The listing builds one solid part. Answer for the finished solid, in the listing's coordinates (mm). A direction names the side the tool comes from. Coordinates: 2 decimals unless noted, no trailing zeros. Order: outer loops, then holes, each group sorted by start corner. A loop starts at its lowest first (then second) coordinate and runs counter-clockwise, first axis right, second up. Notation, with made-up numbers: (-34, 5) - (-18, 5) arc R9 cw to (-18, 21) - close; hole circle Ø11 at (77, 6.25). An arc over 180 degrees is marked (long way). Use a Markdown table: item, result. Add a question column.
Item 1: The mould has two halves that part along Z. Classify faces 1 (the cylindrical face through (37, -3, 0)), 2 (the flat face through (0, 3.3, 0.1)), 3 (the flat face through (-4.411, 1.268, 2.155)): released by +Z, released by -Z, zero draft, split by the parting line, or undercut.
Item 2: The part is cut by section A-A, the plane x = 19. Give the vertices of the cut face in (y, z).
Item 3: Flat-ended cylindrical pins translate along their axes: P1, Ø1, axis at x = 54, z = -2.5, coming from the -Y side; P2, Ø4, axis at x = 3.5, y = -0.5, coming from the -Z side; P3, Ø3, axis at x = 66, y = 3, coming from the -Z side. Find the tip coordinate at first contact, or state that the pin passes through.
Item 4: For faces 4 (the flat face through (75, 0, 0)), 5 (the flat face through (-4, -2.5, 0)), determine the directions among +Z, -Z, +X, -X, +Y, -Y from which every point of the face is accessible in a straight line to the end or side of a thin tool.
Item 5: Find the intervals of material crossed by line 1 along X through (y, z) = (3, 1.5); line 2 along Z through (x, y) = (35, 0); line 3 along Z through (x, y) = (41.5, 2.25), in increasing order.
Autodesk Inventor part; units mm, degrees
ref_plane "Work Plane1" through (29, 0, 0) normal (0, -1, 0) x (1, 0, 0)
ref_plane "YZ Plane" through (0, 0, 0) normal (1, 0, 0) x (0, 1, 0)
ref_plane "XZ Plane" through (0, 0, 0) normal (0, 1, 0) x (-1, 0, 0)
sketch "Sketch1" plane through (0, 0, 0) normal (0, 0, 1) x (1, 0, 0)
  line L0 (-1.3333, 0) -> (75, 0)
  line L1 (75, 0) -> (75, 3)
  line L2 (75, 3) -> (51, 3)
  line L3 (51, 3) -> (50.3865, 3)
  line L4 (50.3865, 3) -> (0, 3)
  line L5 (0, 3) -> (0, 5)
  line L6 (0, 5) -> (-6, 5)
  line L7 (-6, 5) -> (-6, 2.8868)
  line L8 (-6, 2.8868) -> (-3, 2.8868)
  line L9 (-3, 2.8868) -> (-1.3333, 0)
  line L10 (-22.2, 0) -> (91.2, 0)
  line L11 (0, -1) -> (0, 6)
  line L12 (51, 3) -> (0, 3) construction
  dimension "d1" = 24
  dimension "d2" = 0.6136
  dimension "d3" = 6
  dimension "d4" = 3
  dimension "d5" = 60
  dimension "d6" = 6
  dimension "d7" = 6
  dimension "d8" = 5.7735
  dimension "d9" = 10
  dimension "d26" = 75
revolve "Body" add sketch "Sketch1" angle 360 about axis through (-1.3333, 0, 0) along (1, 0, 0)
sketch "Sketch2" plane through (-6, 0, 0) normal (-1, 0, 0) x (0, 0, 1)
  circle A0 centre (0, 0) radius 2.8868
  line L0 (0, -7) -> (0, 7)
  line L1 (-7, 0) -> (7, 0)
  line L2 (2.8868, 0) -> (1.4434, -2.5)
  line L3 (1.4434, -2.5) -> (-1.4434, -2.5)
  line L4 (-1.4434, -2.5) -> (-2.8868, 0)
  line L5 (-2.8868, 0) -> (-1.4434, 2.5)
  line L6 (-1.4434, 2.5) -> (1.4434, 2.5)
  line L7 (1.4434, 2.5) -> (2.8868, 0)
extrude "Slot" add sketch "Sketch2" against normal up to next contours L7 A0 | A0 L2 | L6 L0 A0 | A0 L0 L3 | L0 L6 A0 | A0 L3 L0 | L4 A0 | A0 L5
fillet "Fillet1" radius 0.4 1 edges at (-6, -5, 0)
thread "Thread"
chamfer "Chamfer1" distance 0.6135 distance2 0.6135 1 edges at (75, -3, 0) measured on face at (75, -0.9709, -1.4067)
ref_plane "Work Plane1" through (29, 0, 0) normal (0, -1, 0) x (1, 0, 0)
fillet "Fillet2" radius 0.1 1 edges at (0, -3, 0)
equation "\"d1\" = GEL"
equation "\"d3\" = KOH"
equation "\"d4\" = INTI"
equation "\"d6\" = GD"
equation "\"d7\" = BDM"
equation "\"d8\" = 1.1547 * SW"
equation "\"d9\" = KOD"
equation "\"d26\" = NLG"
equation "\"d30\" = R"
equation "\"d17\" = RR"
equation "\"d13\" = GEL"
equation "\"d15\" = -0.5 * SPD + 0.5 * GD"
equation "\"d16\" = GUL"
equation "\"GD\" = NND"
equation "\"NLG\" = 75"
equation "\"GEL\" = 24"
equation "\"KOD\" = 10"
equation "\"KOH\" = NND"
equation "\"INTI\" = 3"
equation "\"GAL\" = 0.61345 * PTC"
equation "\"GUL\" = 0.61345 * PTC"
equation "\"BDM\" = NND"
equation "\"SW\" = 5"
equation "\"RR\" = 0.4"
equation "\"SPD\" = NND - 1.2269 * PTC"
equation "\"R\" = 0.1"
equation "\"PHH\" = 0.1 * NND"
equation "\"GD1\" = THREADDIA - 1.2269 * PTC"
equation "\"THREADDIA\" = 6"
equation "\"FAWI\" = 45deg"
equation "\"PTC\" = 1"
equation "\"NND\" = 6"
equation "\"FAWI1\" = 30deg"
equation "\"TOA\" = 30deg"
equation "\"E0\" = 1.155 * SW"
properties part number "Unbrako - M6 x 75" material "Steel, Mild"
Solution:
| question | item | result |
|---|---|---|
| 1 | face 1 | split by the parting line |
| 1 | face 2 | zero draft |
| 1 | face 3 | undercut |
| 2 | outline | circle Ø6 at (0, 0) |
| 3 | P1 | stops at y = -2.24 |
| 3 | P2 | stops at z = -3 |
| 3 | P3 | stops at z = -2.6 |
| 4 | face 4 | +Z, -Z, +X, +Y, -Y |
| 4 | face 5 | -X |
| 5 | line 1 | x = -6 to 0 |
| 5 | line 2 | z = -3 to 3 |
| 5 | line 3 | z = -1.98 to 1.98 |
